Autodesk Inventor part; units mm, degrees
ref_plane "YZ Plane" through (0, 0, 0) normal (1, 0, 0) x (0, 1, 0)
ref_plane "XZ Plane" through (0, 0, 0) normal (0, 1, 0) x (-1, 0, 0)
ref_plane "XY Plane" through (0, 0, 0) normal (0, 0, 1) x (1, 0, 0)
sketch "Sketch1" plane through (0, 0, 0) normal (0, 0, 1) x (1, 0, 0)
  line L0 (0, 0) -> (50, 0)
  line L1 (50, 0) -> (50, 70)
  line L2 (50, 70) -> (0, 70)
  line L3 (0, 70) -> (0, 0)
  dimension "d0" = 50
  dimension "d1" = 70
extrude "Extrusion1" add sketch "Sketch1" along normal blind 5
sketch "Sketch2" plane through (0, 0, 5) normal (0, 0, 1) x (1, 0, 0)
  circle A0 centre (7.825, 7) radius 2.5
  circle A1 centre (42.175, 7) radius 2.5
  line L0 (0, 0) -> (50, 0)
  line L1 (50, 0) -> (50, 70)
  line L2 (50, 70) -> (0, 70)
  line L3 (0, 70) -> (0, 0)
  dimension "d4" = 34.35
  dimension "d5" = 5
  dimension "d6" = 5
  dimension "d7" = 50
  dimension "d8" = 7.825
  dimension "d9" = 7
  dimension "d10" = 7
extrude "Extrusion2" cut sketch "Sketch2" against normal up to next contours A0 | A1
sketch "Sketch3" plane through (0, 0, 5) normal (0, 0, 1) x (1, 0, 0)
  circle A0 centre (7.825, 7) radius 2.5
  circle A1 centre (42.175, 7) radius 2.5
  line L0 (0, 0) -> (50, 0)
  line L1 (50, 0) -> (50, 70)
  line L2 (50, 70) -> (0, 70)
  line L3 (0, 70) -> (0, 0)
  line L4 (0, 70) -> (5, 70)
  line L5 (5, 70) -> (5, 35)
  line L6 (5, 35) -> (0, 35)
  line L7 (0, 35) -> (0, 70)
  line L8 (50, 70) -> (45, 70)
  line L9 (45, 70) -> (45, 35)
  line L10 (45, 35) -> (50, 35)
  line L11 (50, 35) -> (50, 70)
  dimension "d13" = 5
  dimension "d14" = 5
  dimension "d15" = 35
extrude "Extrusion3" add sketch "Sketch3" along normal blind 90 contours L3 L2 L5 L6 | L10 L9 L2 L1
sketch "Sketch4" plane through (50, 0, 0) normal (1, 0, 0) x (0, 0, -1)
  line L0 (0, 0) -> (0, 70)
  line L1 (0, 70) -> (-95, 70)
  line L2 (-95, 35) -> (-95, 70)
  line L3 (-5, 35) -> (-95, 35)
  line L4 (-5, 0) -> (-5, 35)
  line L5 (0, 0) -> (-5, 0)
  circle A0 centre (-20, 62.5) radius 2.5
  circle A1 centre (-20, 42.5) radius 2.5
  circle A2 centre (-75, 62.5) radius 2.5
  circle A3 centre (-75, 42.5) radius 2.5
  point P0 (0, 0)
  dimension "d18" = 5
  dimension "d19" = 5
  dimension "d20" = 20
  dimension "d21" = 5
  dimension "d22" = 5
  dimension "d23" = 35
  dimension "d24" = 20
  dimension "d26" = 7.5
  dimension "d27" = 55
  dimension "d28" = 55
  dimension "d31" = 7.5
  dimension "d42" = 20
  dimension "d43" = 20
extrude "Extrusion4" cut sketch "Sketch4" against normal through all contours A0 | A1 | A2 | A3
sketch "Sketch5" plane through (5, 35, 5) normal (1, 0, 0) x (0, 0, -1)
  circle A0 centre (-70, 27.5) radius 2.5
  circle A1 centre (-15, 27.5) radius 2.5
  circle A2 centre (-15, 7.5) radius 2.5
  circle A3 centre (-70, 7.5) radius 2.5
  line L0 (0, 35) -> (0, 0)
  line L1 (0, 35) -> (-90, 35)
  line L2 (-90, 0) -> (-90, 35)
  line L3 (0, 0) -> (-90, 0)
  line L4 (0, 0) -> (-90, 0)
  line L5 (-90, 35) -> (-85, 35)
  line L6 (-85, 35) -> (-85, 0)
  line L7 (-85, 0) -> (-90, 0)
  line L8 (-90, 0) -> (-90, 35)
  point P0 (5, -35)
  dimension "d34" = 5
extrude "Extrusion5" add sketch "Sketch5" along normal up to next contours L6 L3 L2 L1
sketch "Sketch6" plane through (0, 0, 95) normal (0, 0, 1) x (1, 0, 0)
  line L0 (45, 35) -> (45, 70)
  line L1 (45, 70) -> (5, 70)
  line L2 (5, 70) -> (5, 35)
  line L3 (5, 35) -> (0, 35)
  line L4 (0, 35) -> (0, 0)
  line L5 (0, 0) -> (50, 0)
  line L6 (50, 0) -> (50, 35)
  line L7 (50, 35) -> (45, 35)
  circle A0 centre (7.825, 7) radius 2.5
  circle A1 centre (42.175, 7) radius 2.5
  line L8 (50, 70) -> (0, 70)
  line L9 (0, 70) -> (0, 35)
  line L10 (0, 35) -> (50, 35)
  line L11 (50, 35) -> (50, 70)
  line L12 (5, 65) -> (45, 65)
  line L13 (45, 65) -> (45, 40)
  line L14 (45, 40) -> (5, 40)
  line L15 (5, 40) -> (5, 65)
  dimension "d37" = 5
  dimension "d38" = 5
extrude "Extrusion6" cut sketch "Sketch6" against normal through all contours L14 L2 L12 L0
fillet "Fillet1" radius 3 16 edges at (45, 37.5, 5) (5, 37.5, 5) (5, 65, 2.5) (5, 67.5, 5) (5, 65, 92.5) (5, 67.5, 90) (45, 67.5, 5) (45, 65, 2.5) (45, 65, 92.5) (45, 67.5, 90) (45, 40, 2.5) (5, 40, 2.5) (45, 40, 92.5) (45, 37.5, 90) (5, 40, 92.5) (5, 37.5, 90)
sketch "Sketch7" plane through (0, 0, 0) normal (0, 0, -1) x (-1, 0, 0)
  line L0 (-42, 40) -> (-8, 40)
  arc A0 (-8, 40) -> (-5, 43) centre (-8, 43) ccw
  line L1 (-5, 43) -> (-5, 62)
  arc A1 (-5, 62) -> (-8, 65) centre (-8, 62) ccw
  line L2 (-8, 65) -> (-42, 65)
  arc A2 (-42, 65) -> (-45, 62) centre (-42, 62) ccw
  line L3 (-45, 62) -> (-45, 43)
  arc A3 (-45, 43) -> (-42, 40) centre (-42, 43) ccw
  line L4 (-50, 70) -> (0, 70)
  line L5 (0, 70) -> (0, 35)
  line L6 (0, 35) -> (-50, 35)
  line L7 (-50, 35) -> (-50, 70)
  line L8 (-8, 40) -> (-42, 40)
  arc A4 (-45, 43) -> (-42, 40) centre (-42, 43) ccw
  line L9 (-45, 43) -> (-45, 62)
  arc A5 (-42, 65) -> (-45, 62) centre (-42, 62) ccw
  line L10 (-42, 65) -> (-8, 65)
  arc A6 (-5, 62) -> (-8, 65) centre (-8, 62) ccw
  line L11 (-5, 62) -> (-5, 43)
  arc A7 (-8, 40) -> (-5, 43) centre (-8, 43) ccw
  circle A8 centre (-7.825, 7) radius 2.5
  circle A9 centre (-42.175, 7) radius 2.5
  line L12 (0, 0) -> (-50, 0)
  line L13 (0, 70) -> (0, 0)
  line L14 (-50, 70) -> (0, 70)
  line L15 (-50, 0) -> (-50, 70)
  line L16 (-5, 43) -> (-5, 62)
  line L17 (-5, 43) -> (-45, 43)
  line L18 (-45, 43) -> (-45, 14)
  line L19 (-45, 14) -> (-5, 14)
  line L20 (-5, 14) -> (-5, 43)
  line L21 (-45, 43) -> (-45, 62)
  dimension "d44" = 7
  dimension "d45" = 7
extrude "Extrusion7" cut sketch "Sketch7" against normal up to next contours L0 A0 L20 L6 L18 A3 | L6 L20 L19 L18
fillet "Fillet2" radius 20 1 edges at (2.5, 35, 5)
fillet "Fillet3" radius 5 2 edges at (5, 14, 2.5) (45, 14, 2.5)
equation "\"d8\" = -0.5 * d4 + 0.5 * d7"
equation "\"d10\" = d9"
equation "\"d13\" = d14"
equation "\"d26\" = -0.5 * d24 + 0.5 * d23"
equation "\"d28\" = d27"
equation "\"d31\" = d26"
equation "\"d43\" = d42"
equation "\"d45\" = d44"
properties part number "tubing_alignment_arm[2]"
Verification items for the finished model (mm, model axes). A direction names the side the tool comes from. Give positions to 0.01 mm unless a question says otherwise; leave off trailing zeros. Loops run counter-clockwise (first coordinate to the right, second up) from the corner with the lowest first, then second, coordinate; pieces in that order, holes last. Notation, with made-up numbers: M 25.25,-28 L 53.25,-28 A20 cw 53.25,1 Z; hole C -39,82 d11. An arc over 180 degrees is marked long. One line per question, with ' | ' between items.
Item 1: Draft check along Z on faces 1 (the face through (25, 68, 90)), 2 (the face through (25, 14, 2)), 3 (the face through (5.9, 66.83, 89.14)), 4 (the face through (25, 37, 95)). Enter one of: +Z half, -Z half, draft (parallel to the pull), parting line (faces both ways), or undercut.
Completed:
face 1: undercut | face 2: draft | face 3: undercut | face 4: +Z half
Item 2: Section check C-C, the plane x = 30. Record the cut outline in (y, z).
Completed:
outline: M 0,0 L 14,0 L 14,5 L 0,5 Z; M 35,90 L 40,90 L 40,95 L 35,95 Z; M 65,0 L 70,0 L 70,5 L 65,5 Z; M 65,90 L 70,90 L 70,95 L 65,95 Z
Item 3: Depth check by flat-ended pin: P1, Ø3, axis at y = 62.5, z = 20, coming from the +X side; P2, Ø5.5, axis at x = 27, z = 93, coming from the -Y side; P3, Ø7.5, axis at x = 15.5, y = 11, coming from the +Z side. Enter the tip coordinate at first touch or a pass-through.
Completed:
P1: passes through | P2: stops at y = 35 | P3: stops at z = 5
Item 4: Thickness scan on line 1 (Y direction, x = 48, z = 75); line 2 (Z direction, x = 3.05, y = 42.5); line 3 (X direction, y = 41, z = 70). Record the ranges inside material, lowest first. Write a range as [from, to].
Completed:
line 1: y = [35, 40], [45, 60], [65, 70] | line 2: z = [0, 17.5], [22.5, 72.5], [77.5, 95] | line 3: x = [0, 5], [45, 50]
Item 5: Section check D-D, the plane z = 42. Record the cut outline in (x, y).
Completed:
outline: M 0,35 L 5,35 L 5,70 L 0,70 Z; M 45,35 L 50,35 L 50,70 L 45,70 Z
Item 6: Tool access check on faces 5 (the face through (25, 68, 5)), 6 (the face through (4.5, 70, 50.8)), 7 (the face through (45, 51, 47)), 8 (the face through (25, 65, 93)), 9 (the face through (25, 0, 2)). Record the directions out of +Z, -Z, +X, -X, +Y, -Y that give a thin tool (end or side, any length) a straight path to the whole face; none if there is none.
Completed:
face 5: +Y, -Y | face 6: +Z, -Z, +X, -X, +Y | face 7: none | face 8: +Z, -Z | face 9: +Z, -Z, +X, -X, -Y
Item 7: Section check A-A, the plane y = 7. Record the cut outline in (x, z) (3 decimals).
Completed:
outline: M 0,0 L 5.325,0 L 5.325,5 L 0,5 Z; M 10.325,0 L 39.675,0 L 39.675,5 L 10.325,5 Z; M 44.675,0 L 50,0 L 50,5 L 44.675,5 Z
Item 8: Section check B-B, the plane z = 75. Record the cut outline in (x, y).
Completed:
outline: M 0,35 L 5,35 L 5,40 L 0,40 Z; M 0,45 L 5,45 L 5,60 L 0,60 Z; M 0,65 L 5,65 L 5,70 L 0,70 Z; M 45,35 L 50,35 L 50,40 L 45,40 Z; M 45,45 L 50,45 L 50,60 L 45,60 Z; M 45,65 L 50,65 L 50,70 L 45,70 Z
